```python
from build123d import *

# Parameters (mm, degrees)
F0_R     = 1.1
F1_DEPTH = 1
F3_DEPTH = 10
F4_R     = 2.5
F5_DEPTH = 1
F6_R     = 0.7
F7_DEPTH = 0.5
F8_R     = 0.49999
F9_SIZE  = 0.5
F10_SIZE = 0.1
F11_SIZE = 0.2


# Not quite as in the source:
# - a fillet or chamfer is up to 0.001 mm smaller than in the source, because OpenCascade refuses the exact size


with BuildPart() as f1:
    # F0 (on Top) → F1 (new body)
    with BuildSketch(Plane.XY):
        with BuildLine():
            ThreePointArc((-10.5473609378, 1.9236413397), (-12, 0), (-10.5473609378, -1.9236413397))
            Line((-10.5473609378, -1.9236413397), (-6.7646138101, -3))
            ThreePointArc((-6.7646138101, -3), (0, -7.4), (6.7646138101, -3))
            Line((6.7646138101, -3), (10.5473609378, -1.9236413397))
            ThreePointArc((10.5473609378, -1.9236413397), (12, 0), (10.5473609378, 1.9236413397))
            Line((10.5473609378, 1.9236413397), (6.7646138101, 3))
            ThreePointArc((6.7646138101, 3), (0, 7.4), (-6.7646138101, 3))
            Line((-6.7646138101, 3), (-10.5473609378, 1.9236413397))
        make_face()
        with Locations((-10, 0)):
            Circle(F0_R, mode=Mode.SUBTRACT)
        with Locations((10, 0)):
            Circle(F0_R, mode=Mode.SUBTRACT)
    extrude(amount=F1_DEPTH)

    # F2 (on face) → F3 (join)
    with BuildSketch(Plane.XY.offset(1)):
        with BuildLine():
            ThreePointArc((6.7646138101, -3), (7.2394109634, -1.5332739164), (7.4, 0))
            ThreePointArc((7.4, 0), (7.2394109634, 1.5332739164), (6.7646138101, 3))
            ThreePointArc((6.7646138101, 3), (0, 7.4), (-6.7646138101, 3))
            ThreePointArc((-6.7646138101, 3), (-7.4, 0), (-6.7646138101, -3))
            ThreePointArc((-6.7646138101, -3), (0, -7.4), (6.7646138101, -3))
        make_face()
    extrude(amount=F3_DEPTH)

    # F4 (on face) → F5 (join)
    with BuildSketch(Plane.XY.offset(11)):
        Circle(F4_R)
    extrude(amount=F5_DEPTH)

    # F6 (on face) → F7 (join)
    with BuildSketch(Plane.XY.offset(12)):
        Circle(F6_R)
    extrude(amount=F7_DEPTH)

    # F8 (radius 0.5 in the source; OpenCascade refuses exactly that, so slightly less here)
    f8_edges = [f1.edges().sort_by_distance(p)[0] for p in [
        (-0.7, 0, 12.5),
    ]]
    fillet(f8_edges, radius=F8_R)

    # F9
    f9_edges = [f1.edges().sort_by_distance(p)[0] for p in [
        (-7.4, 0, 11),
    ]]
    chamfer(f9_edges, length=F9_SIZE)

    # F10
    f10_edges = [f1.edges().sort_by_distance(p)[0] for p in [
        (-8.655987, 2.461821, 0),
        (-12, 0, 0),
        (-8.655987, -2.461821, 0),
        (0, -7.4, 0),
        (8.655987, -2.461821, 0),
        (12, 0, 0),
        (8.655987, 2.461821, 0),
        (0, 7.4, 0),
        (-11.1, 0, 0),
        (8.9, 0, 0),
    ]]
    chamfer(f10_edges, length=F10_SIZE)

    # F11
    f11_edges = [f1.edges().sort_by_distance(p)[0] for p in [
        (-2.5, 0, 12),
    ]]
    chamfer(f11_edges, length=F11_SIZE)


solid = f1.part
```
Build history of the part. All positions in model axes, mm. A direction names the side the tool comes from. Coordinates: 2 decimals unless noted, no trailing zeros. Order: outer loops, then holes, each group sorted by start corner. A loop starts at its lowest first (then second) coordinate and runs counter-clockwise, first axis right, second up. Notation, with made-up numbers: M 74,73 L 96,73 A32 ccw 96,105 Z; hole C 37,73 d9. An arc over 180 degrees is marked long. One line per question, with ' | ' between items. Start each with the question number.
1. Cut at A-A (z = 8.5). Write the cut outline in (x, y), plus the area to 3 significant figures.
2. Cut at B-B (x = -10). Write the cut outline in (y, z).
3. Wall check: line 1 along Z through (x, y) = (-8.25, -0.75); line 2 along Z through (x, y) = (-4.75, 4.5); line 3 along Y through (x, z) = (10, 0.75). Give the ranges that are in metal, low to high. Write a range as [from, to].
4. Flat gauge pins, fed straight in: P1, Ø5, axis at y = 0, z = 6.5, coming from the +X side; P2, Ø1.5, axis at y = -5.5, z = 11, coming from the +X side; P3, Ø2.5, axis at x = -10, y = 0, coming from the +Z side; P4, Ø1.5, axis at x = 9.5, y = 3.5, coming from the -Z side. Where does each tip first touch, or does it go through?
5. Tool access for faces 5 (the face through (-0.54, -2.44, 11.39)), 6 (the face through (-12, 0, 0.5)): list every direction of +Z, -Z, +X, -X, +Y, -Y with a clear straight run to the whole face (end or side of a thin tool).
6. Mould opens along Y. For faces 1 (the face through (8.63, -2.47, 0.54)), 2 (the face through (-8.984, -0.421, 0.544)), 3 (the face through (8.682, 2.454, 0.544)), 4 (the face through (12, 0, 0.5)) say: +Y half, -Y half, draft (parallel to the pull), parting line (faces both ways), or undercut.
The answers:
1) outline: C 0,0 d14.8 | area: 172 mm2
2) outline: M -2.08,0.1 L -1.98,0 L -1.2,0 L -1.1,0.1 L -1.1,1 L -2.08,1 Z; M 1.1,0.1 L 1.2,0 L 1.98,0 L 2.08,0.1 L 2.08,1 L 1.1,1 Z
3) line 1: z = [0, 1] | line 2: z = [0, 11] | line 3: y = [-2.08, -1.1], [1.1, 2.08]
4) P1: stops at x = 7.4 | P2: stops at x = 5.51 | P3: stops at z = 1 | P4: passes through
5) face 5: +Z | face 6: +Z, -Z, -X
6) face 1: -Y half | face 2: undercut | face 3: +Y half | face 4: parting line
